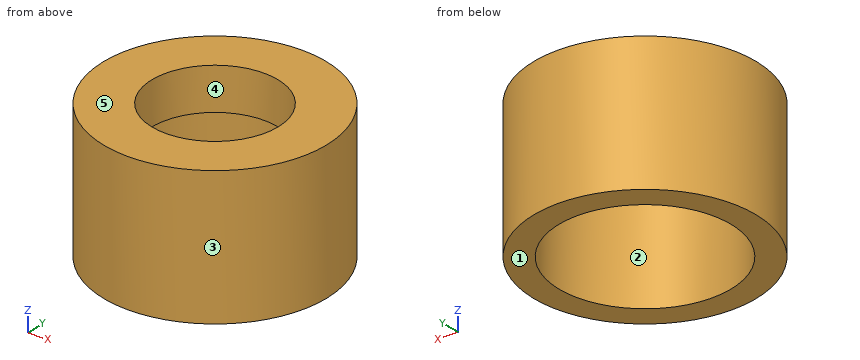
```python
from build123d import *

# Parameters (mm, degrees)
SKETCH1_R           = 13.462
BOSS_EXTRUDE3_DEPTH = 16.51
SKETCH1_15_R        = 7.62
CUT_EXTRUDE3_DEPTH  = 16.51
SKETCH1_16_R        = 10.414
SKETCH1_16_R_2      = 7.62
CUT_EXTRUDE4_DEPTH  = 11.43


with BuildPart() as part:
    # Sketch1 → Boss-Extrude3 (new body)
    with BuildSketch(Plane.XY):
        Circle(SKETCH1_R)
    extrude(amount=BOSS_EXTRUDE3_DEPTH)

    # Sketch1<15> → Cut-Extrude3 (cut)
    with BuildSketch(Plane.XY):
        Circle(SKETCH1_15_R)
    extrude(amount=CUT_EXTRUDE3_DEPTH, mode=Mode.SUBTRACT)

    # Sketch1<16> → Cut-Extrude4 (cut)
    with BuildSketch(Plane.XY):
        Circle(SKETCH1_16_R)
        Circle(SKETCH1_16_R_2, mode=Mode.SUBTRACT)
    extrude(amount=CUT_EXTRUDE4_DEPTH, mode=Mode.SUBTRACT)


solid = part.part
```
Could you check a few things on this model? Use its own coordinates, in mm. Face numbers are marked on the shaded views. A direction names the side the tool comes from. Round coordinates to 2 decimals unless told otherwise and drop trailing zeros. Loops run counter-clockwise (first coordinate to the right, second up) from the corner with the lowest first, then second, coordinate; pieces in that order, holes last. Notation, with made-up numbers: M -1,87.5 L 21,87.5 A28 cw 21,117.5 Z; hole C 67,-39.5 d9. An arc over 180 degrees is marked long. Write item = value, one per line.
1. I want a section at C-C, the plane z = 14. Write out the boundary of the cut face in (x, y), and give its area (3 significant figures).
Results below:
outline = C 0,0 d26.92; hole C 0,0 d15.24
area = 387 mm²
2. I need wall thicknesses on probe 1 along Y at (x, z) = (0, 6.5); probe 2 along Y at (x, z) = (0, 12.25); probe 3 along X at (y, z) = (2.75, 4). Which ranges of each line are inside material? Lowest first, please.
Results below:
probe_1 = -13.46 to -10.41, 10.41 to 13.46
probe_2 = -13.46 to -7.62, 7.62 to 13.46
probe_3 = -13.18 to -10.04, 10.04 to 13.18
3. I want a section at D-D, the plane y = 10. Write out the boundary of the cut face in (x, z).
Results below:
outline = M -9.01,0 L -2.91,0 L -2.91,11.43 L 2.91,11.43 L 2.91,0 L 9.01,0 L 9.01,16.51 L -9.01,16.51 Z
4. Thinking about a two-plate mould opening in Y: for the marked faces 3, 4 and 5, which applies, +Y half, -Y half, draft (parallel to the pull), parting line (faces both ways), or undercut?
Results below:
face_3 = parting line
face_4 = undercut
face_5 = draft
5. Will these pins go through, and if not, where does the flat tip stop? P1, Ø5, axis at x = -6.5, y = -4, coming from the -Z side; P2, Ø4, axis at y = -8.5, z = 12, coming from the -X side; P3, Ø12.5, axis at x = 0, y = 0, coming from the +Z side; P4, Ø6, axis at x = 6.5, z = 13, coming from the -Y side.
Results below:
P1 = 11.43
P2 = -11.79
P3 = through
P4 = -13
6. Which directions (+Z, -Z, +X, -X, +Y, -Y) give clear straight access to the entire face, cutting with the end or side of a thin tool? Please do the marked faces 1 and 2.
Results below:
face_1 = -Z, +X, -X, +Y, -Y
face_2 = -Z
7. I want a section at A-A, the plane y = 0. Write out the boundary of the cut face in (x, z).
Results below:
outline = M -13.46,0 L -10.41,0 L -10.41,11.43 L -7.62,11.43 L -7.62,16.51 L -13.46,16.51 Z; M 7.62,11.43 L 10.41,11.43 L 10.41,0 L 13.46,0 L 13.46,16.51 L 7.62,16.51 Z
